Geometry: final body of the model. Coordinates: model frame, mm. Coordinates: 2 decimals unless noted, no trailing zeros. Order: outer loops, then holes, each group sorted by start corner. A loop starts at its lowest first (then second) coordinate and runs counter-clockwise, first axis right, second up. Notation, with made-up numbers: (65.5, -16.75) -> (111.5, -16.75) arc R19 cw to (111.5, 19.25) -> close; hole circle Ø4 at (-33.5, -27). An arc over 180 degrees is marked (long way). Use CSV: the item, a comma, the result in double quotes. Start each with the question number.
from build123d import *

# Parameters (mm, degrees)
SKETCH_1_R          = 2.1
SKETCH_1_R_2        = 35.6
EXTRUDE_1_DEPTH     = 3
SKETCH_2_R          = 2.1
CUT_EXTRUDE_1_DEPTH = 3
CUT_EXTRUDE_2_DEPTH = 130.653384067


with BuildPart() as part:
    # 草图1 → 凸台-拉伸1 (new body)
    with BuildSketch(Plane.XY):
        with BuildLine():
            Line((0, 49), (115, 49))
            ThreePointArc((115, 49), (118.535533906, 47.535533906), (120, 44))
            Line((120, 44), (120, 24))
            ThreePointArc((120, 24), (118.535533906, 20.464466094), (115, 19))
            Line((115, 19), (79, 19))
            ThreePointArc((79, 19), (77.086582838, 18.619397663), (75.464466094, 17.535533906))
            Line((75.464466094, 17.535533906), (61.464466094, 3.535533906))
            ThreePointArc((61.464466094, 3.535533906), (60, 0), (61.464466094, -3.535533906))
            Line((61.464466094, -3.535533906), (75.464466094, -17.535533906))
            ThreePointArc((75.464466094, -17.535533906), (77.086582838, -18.619397663), (79, -19))
            Line((79, -19), (115, -19))
            ThreePointArc((115, -19), (118.535533906, -20.464466094), (120, -24))
            Line((120, -24), (120, -44))
            ThreePointArc((120, -44), (118.535533906, -47.535533906), (115, -49))
            Line((115, -49), (0, -49))
            ThreePointArc((0, -49), (-49, 0), (0, 49))
        make_face()
        with Locations((-45, 0)):
            Circle(SKETCH_1_R, mode=Mode.SUBTRACT)
        with Locations((-22.5, 38.97114317)):
            Circle(SKETCH_1_R, mode=Mode.SUBTRACT)
        with Locations((22.5, 38.97114317)):
            Circle(SKETCH_1_R, mode=Mode.SUBTRACT)
        with Locations((45, 0)):
            Circle(SKETCH_1_R, mode=Mode.SUBTRACT)
        with Locations((22.5, -38.97114317)):
            Circle(SKETCH_1_R, mode=Mode.SUBTRACT)
        with Locations((-22.5, -38.97114317)):
            Circle(SKETCH_1_R, mode=Mode.SUBTRACT)
        Circle(SKETCH_1_R_2, mode=Mode.SUBTRACT)
    extrude(amount=EXTRUDE_1_DEPTH)

    # 草图2 → 切除-拉伸1 (cut)
    with BuildSketch(Plane.XY):
        with Locations((85, 44)):
            Circle(SKETCH_2_R)
        with Locations((115, 44)):
            Circle(SKETCH_2_R)
        with Locations(Location((115, 24, 0), (0, 0, 180))):
            Circle(SKETCH_2_R)
        with Locations(Location((85, 24, 0), (0, 0, 180))):
            Circle(SKETCH_2_R)
        with Locations((85, -24)):
            Circle(SKETCH_2_R)
        with Locations((115, -24)):
            Circle(SKETCH_2_R)
        with Locations(Location((115, -44, 0), (0, 0, 180))):
            Circle(SKETCH_2_R)
        with Locations(Location((85, -44, 0), (0, 0, 180))):
            Circle(SKETCH_2_R)
    extrude(amount=CUT_EXTRUDE_1_DEPTH, mode=Mode.SUBTRACT)

    # 草图3 → 切除-拉伸2 (cut, through all)
    with BuildSketch(Plane.XY):
        with BuildLine():
            Line((34.394767044, 42), (76, 42))
            ThreePointArc((76, 42), (78.121320344, 41.121320344), (79, 39))
            Line((79, 39), (79, 32.213203436))
            ThreePointArc((79, 32.213203436), (78.771638598, 31.065153139), (78.121320344, 30.091883092))
            Line((78.121320344, 30.091883092), (54.908116908, 6.878679656))
            ThreePointArc((54.908116908, 6.878679656), (53.934846861, 6.228361402), (52.786796564, 6))
            Line((52.786796564, 6), (51.215232109, 6))
            ThreePointArc((51.215232109, 6), (49.28620286, 6.702426029), (48.26050718, 8.480769231))
            ThreePointArc((48.26050718, 8.480769231), (42.740359483, 23.963757452), (32.410453561, 36.75))
            ThreePointArc((32.410453561, 36.75), (31.588524004, 40.060660172), (34.394767044, 42))
        make_face()
        with BuildLine():
            Line((52.786796564, -6), (51.215232109, -6))
            ThreePointArc((51.215232109, -6), (49.28620286, -6.702426029), (48.26050718, -8.480769231))
            ThreePointArc((48.26050718, -8.480769231), (42.740359483, -23.963757452), (32.410453561, -36.75))
            ThreePointArc((32.410453561, -36.75), (31.588524004, -40.060660172), (34.394767044, -42))
            Line((34.394767044, -42), (76, -42))
            ThreePointArc((76, -42), (78.121320344, -41.121320344), (79, -39))
            Line((79, -39), (79, -32.213203436))
            ThreePointArc((79, -32.213203436), (78.771638598, -31.065153139), (78.121320344, -30.091883092))
            Line((78.121320344, -30.091883092), (54.908116908, -6.878679656))
            ThreePointArc((54.908116908, -6.878679656), (53.934846861, -6.228361402), (52.786796564, -6))
        make_face()
        with BuildLine():
            Line((93, 26), (107, 26))
            ThreePointArc((107, 26), (109.121320344, 26.878679656), (110, 29))
            Line((110, 29), (110, 39))
            ThreePointArc((110, 39), (109.121320344, 41.121320344), (107, 42))
            Line((107, 42), (93, 42))
            ThreePointArc((93, 42), (90.878679656, 41.121320344), (90, 39))
            Line((90, 39), (90, 29))
            ThreePointArc((90, 29), (90.878679656, 26.878679656), (93, 26))
        make_face()
        with BuildLine():
            Line((110, -29), (110, -39))
            ThreePointArc((110, -39), (109.121320344, -41.121320344), (107, -42))
            Line((107, -42), (93, -42))
            ThreePointArc((93, -42), (90.878679656, -41.121320344), (90, -39))
            Line((90, -39), (90, -29))
            ThreePointArc((90, -29), (90.878679656, -26.878679656), (93, -26))
            Line((93, -26), (107, -26))
            ThreePointArc((107, -26), (109.121320344, -26.878679656), (110, -29))
        make_face()
    extrude(amount=CUT_EXTRUDE_2_DEPTH, mode=Mode.SUBTRACT)


solid = part.part
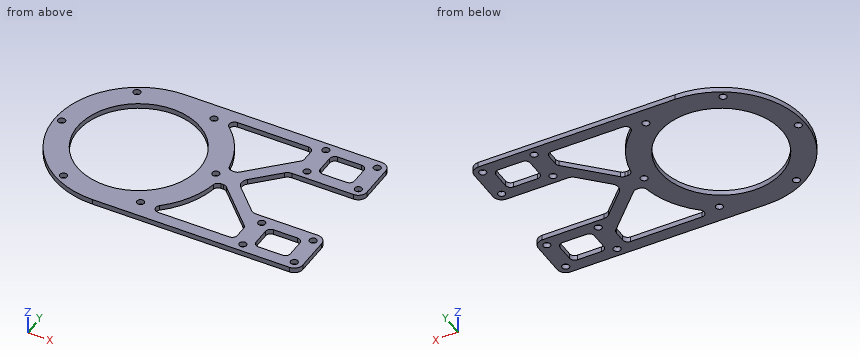
(1) Section A-A (x = 97). Return loops of the section in (y, z), then the cut area to 3 significant figures.
(2) Section C-C (x = -2). Return loops of the section in (y, z).
(3) Section D-D (z = 1.15). State how many separate pieces and enclosed holes the cut face has, then the cut area to 3 significant figures.
(4) First-contact query: pin 1 (1.5 mm diameter, centred on y = -37, z = 1.5, fed in from -X). Flat tip, straight axial feed; report the tip coordinate or a pass-through.
(5) Section B-B (y = 0). Return loops of the section in (x, z).
(6) Line query: line 1 (Y direction, x = 102.5, z = 1.8); line 2 (Y direction, x = 85, z = 1.3); line 3 (Y direction, x = 0, z = 2.5). Output: solid intervals per line, ascending. Write a range as from..to.
Check sheet entries:
1,outline,"(-49, 0) -> (-42, 0) -> (-42, 3) -> (-49, 3) -> close; (-26, 0) -> (-19, 0) -> (-19, 3) -> (-26, 3) -> close; (19, 0) -> (26, 0) -> (26, 3) -> (19, 3) -> close; (42, 0) -> (49, 0) -> (49, 3) -> (42, 3) -> close"
1,area,"84.0 mm^2"
2,outline,"(-48.96, 0) -> (-35.54, 0) -> (-35.54, 3) -> (-48.96, 3) -> close; (35.54, 0) -> (48.96, 0) -> (48.96, 3) -> (35.54, 3) -> close"
3,separate pieces,"1"
3,enclosed holes,"19"
3,area,"6,640 mm^2"
4,pin 1,"stops at x = -32.97"
5,outline,"(-49, 0) -> (-47.1, 0) -> (-47.1, 3) -> (-49, 3) -> close; (-42.9, 0) -> (-35.6, 0) -> (-35.6, 3) -> (-42.9, 3) -> close; (35.6, 0) -> (42.9, 0) -> (42.9, 3) -> (35.6, 3) -> close; (47.1, 0) -> (60, 0) -> (60, 3) -> (47.1, 3) -> close"
6,line 1,"y = -49..-42, -26..-19, 19..26, 42..49"
6,line 2,"y = -49..-46.1, -41.9..-26.1, -21.9..-19, 19..21.9, 26.1..41.9, 46.1..49"
6,line 3,"y = -49..-35.6, 35.6..49"
